Geometry check sheet. Reference: the model listing, model coordinates, mm. A direction names the side the tool comes from. Give positions to 0.01 mm unless a question says otherwise; leave off trailing zeros. Loops run counter-clockwise (first coordinate to the right, second up) from the corner with the lowest first, then second, coordinate; pieces in that order, holes last. Notation, with made-up numbers: (88, -34) -> (146, -34) arc R21 ccw to (146, -12) -> close; hole circle Ø5 at (47, 41). An arc over 180 degrees is marked (long way). One line per question, with ' | ' between items.
from build123d import *

# Parameters (mm, degrees)
SKETCH_1_W      = 38
SKETCH_1_H      = 38
SKETCH_1_R      = 1.25
EXTRUDE_1_DEPTH = 1.5
SKETCH_2_W      = 16
SKETCH_2_H      = 16
EXTRUDE_2_DEPTH = 7
SKETCH_3_R      = 7.5
EXTRUDE_3_DEPTH = 7
EXTRUDE_4_DEPTH = 3
SKETCH_6_W      = 10
SKETCH_6_H      = 5
EXTRUDE_5_DEPTH = 15
SKETCH_7_R      = 7
EXTRUDE_6_DEPTH = 10
SKETCH_8_W      = 8
SKETCH_8_H      = 1
EXTRUDE_7_DEPTH = 2


with BuildPart() as part:
    # 草图1 → 凸台-拉伸1 (new body)
    with BuildSketch(Plane.XY):
        Rectangle(SKETCH_1_W, SKETCH_1_H)
        with Locations((-14, 14)):
            Circle(SKETCH_1_R, mode=Mode.SUBTRACT)
        with Locations((14, 14)):
            Circle(SKETCH_1_R, mode=Mode.SUBTRACT)
        with Locations((14, -14)):
            Circle(SKETCH_1_R, mode=Mode.SUBTRACT)
        with Locations((-14, -14)):
            Circle(SKETCH_1_R, mode=Mode.SUBTRACT)
    extrude(amount=EXTRUDE_1_DEPTH)

    # 草图2 → 凸台-拉伸2 (add)
    with BuildSketch(Plane.XY.offset(1.5)):
        Rectangle(SKETCH_2_W, SKETCH_2_H)
    extrude(amount=EXTRUDE_2_DEPTH)

    # 草图3 → 凸台-拉伸3 (add)
    with BuildSketch(Plane.XY.offset(8.5)):
        Circle(SKETCH_3_R)
    extrude(amount=EXTRUDE_3_DEPTH)

    # 草图5 → 凸台-拉伸4 (add)
    with BuildSketch(Plane.XY.offset(1.5)):
        with BuildLine():
            Line((10, -2), (-10, -2))
            ThreePointArc((-10, -2), (-12, 0), (-10, 2))
            Line((-10, 2), (10, 2))
            ThreePointArc((10, 2), (12, 0), (10, -2))
        make_face()
    extrude(amount=EXTRUDE_4_DEPTH)

    # 草图6 → 凸台-拉伸5 (add)
    with BuildSketch(Plane(origin=(0, 0, 0), x_dir=(-1, 0, 0), z_dir=(0, 0, -1))):
        with Locations((-5, 13.5)):
            Rectangle(SKETCH_6_W, SKETCH_6_H)
    extrude(amount=EXTRUDE_5_DEPTH)

    # 草图7 → 凸台-拉伸6 (add)
    with BuildSketch(Plane.XY.offset(15.5)):
        Circle(SKETCH_7_R)
    extrude(amount=EXTRUDE_6_DEPTH)

    # 草图8 → 凸台-拉伸7 (add)
    with BuildSketch(Plane.XY.offset(1.5)):
        with Locations((5, 13.5)):
            Rectangle(SKETCH_8_W, SKETCH_8_H)
    extrude(amount=EXTRUDE_7_DEPTH)


solid = part.part
Item 1: Sectioned sample at D-D (y = 10). Record the cut outline in (x, z), plus the area to 3 significant figures.
Result:
outline: (-19, 0) -> (19, 0) -> (19, 1.5) -> (-19, 1.5) -> close | area: 57.0 mm2
Item 2: Scan lines: probe 1 along Y at (x, z) = (-14, 0.6); probe 2 along Z at (x, y) = (11, 4); probe 3 along Z at (x, y) = (0.5, 6). Record each from-to range of solid material in increasing order.
Result:
probe 1: -19 to -15.25, -12.75 to 12.75, 15.25 to 19 | probe 2: 0 to 1.5 | probe 3: 0 to 25.5
Item 3: Release check for a two-part mould opening along X. For faces 1 (the face through (7, 2, 15.5)), 2 (the face through (-14.16, 15.24, 0.74)), 3 (the face through (10, 13, -7)), 4 (the face through (-12, 0, 3)) record: pulls with the +X half, pulls with the -X half, needs draft (parallel to the pull), parting line crosses it, or undercut.
Result:
face 1: needs draft | face 2: undercut | face 3: pulls with the +X half | face 4: pulls with the -X half
Item 4: Depth check by flat-ended pin: pin 1 Ø0.6 at (x, z) = (6, 2) entering from -Y; pin 2 Ø4 at (y, z) = (6.5, 7) entering from -X; pin 3 Ø4.5 at (x, y) = (-9.5, 0.5) entering from +Z. Enter the tip coordinate at first touch or a pass-through.
Result:
pin 1: y = -8 | pin 2: x = -8 | pin 3: z = 15.5
Item 5: Set-up check for faces 5 (the face through (9, -2, 3)), 6 (the face through (0, 13, -7)), 7 (the face through (-7.493, 0.33, 11.951)), 8 (the face through (5, 16, -7)): record each of +Z, -Z, +X, -X, +Y, -Y from which the full face is reachable in a straight line by a thin tool's end or side.
Result:
face 5: +Z, +X, -Y | face 6: -Z, -X, +Y, -Y | face 7: +Z | face 8: -Z, +X, -X, +Y
Item 6: Sectioned sample at C-C (z = -5.5). Record the cut outline in (x, y), plus the area to 3 significant figures.
Result:
outline: (0, 11) -> (10, 11) -> (10, 16) -> (0, 16) -> close | area: 50.0 mm2
Item 7: Sectioned sample at A-A (x = 14). Record the cut outline in (y, z).
Result:
outline: (-19, 0) -> (-15.25, 0) -> (-15.25, 1.5) -> (-19, 1.5) -> close; (-12.75, 0) -> (12.75, 0) -> (12.75, 1.5) -> (-12.75, 1.5) -> close; (15.25, 0) -> (19, 0) -> (19, 1.5) -> (15.25, 1.5) -> close
